from build123d import *

# Parameters (mm, degrees)
F0_R     = 1.5
F1_DEPTH = 1
F3_DEPTH = 25


with BuildPart() as f1:
    # F0 (on Top) → F1 (new body)
    with BuildSketch(Plane.XY):
        Polygon((125, -216.506351), (250, 0), (125, 216.506351), (-125, 216.506351), (-250, 0), (-125, -216.506351), align=None)
        with Locations((-153.300327, -114.488747)):
            Circle(F0_R, mode=Mode.SUBTRACT)
        with Locations((-22.5, -190.006351)):
            Circle(F0_R, mode=Mode.SUBTRACT)
        with Locations((-22.5, -174.006351)):
            Circle(F0_R, mode=Mode.SUBTRACT)
        with Locations((-139.44392, -106.488747)):
            Circle(F0_R, mode=Mode.SUBTRACT)
        with Locations((-175.800327, -75.517604)):
            Circle(F0_R, mode=Mode.SUBTRACT)
        with Locations((-161.94392, -67.517604)):
            Circle(F0_R, mode=Mode.SUBTRACT)
        with Locations((-66.697786, -64.488747)):
            Circle(F0_R, mode=Mode.SUBTRACT)
        with Locations((-22.5, -90.006351)):
            Circle(F0_R, mode=Mode.SUBTRACT)
        with Locations((-52.84138, -56.488747)):
            Circle(F0_R, mode=Mode.SUBTRACT)
        with Locations((-22.5, -74.006351)):
            Circle(F0_R, mode=Mode.SUBTRACT)
        with Locations((-89.197786, -25.517604)):
            Circle(F0_R, mode=Mode.SUBTRACT)
        with Locations((-75.34138, -17.517604)):
            Circle(F0_R, mode=Mode.SUBTRACT)
        with Locations((22.5, -190.006351)):
            Circle(F0_R, mode=Mode.SUBTRACT)
        with Locations((22.5, -174.006351)):
            Circle(F0_R, mode=Mode.SUBTRACT)
        with Locations((153.300327, -114.488747)):
            Circle(F0_R, mode=Mode.SUBTRACT)
        with Locations((22.5, -90.006351)):
            Circle(F0_R, mode=Mode.SUBTRACT)
        with Locations((22.5, -74.006351)):
            Circle(F0_R, mode=Mode.SUBTRACT)
        with Locations((52.84138, -56.488747)):
            Circle(F0_R, mode=Mode.SUBTRACT)
        with Locations((66.697786, -64.488747)):
            Circle(F0_R, mode=Mode.SUBTRACT)
        with Locations((75.34138, -17.517604)):
            Circle(F0_R, mode=Mode.SUBTRACT)
        with Locations((89.197786, -25.517604)):
            Circle(F0_R, mode=Mode.SUBTRACT)
        with Locations((139.44392, -106.488747)):
            Circle(F0_R, mode=Mode.SUBTRACT)
        with Locations((175.800327, -75.517604)):
            Circle(F0_R, mode=Mode.SUBTRACT)
        with Locations((161.94392, -67.517604)):
            Circle(F0_R, mode=Mode.SUBTRACT)
        with Locations((-161.94392, 67.517604)):
            Circle(F0_R, mode=Mode.SUBTRACT)
        with Locations((-175.800327, 75.517604)):
            Circle(F0_R, mode=Mode.SUBTRACT)
        with Locations((-139.44392, 106.488747)):
            Circle(F0_R, mode=Mode.SUBTRACT)
        with Locations((-89.197786, 25.517604)):
            Circle(F0_R, mode=Mode.SUBTRACT)
        with Locations((-75.34138, 17.517604)):
            Circle(F0_R, mode=Mode.SUBTRACT)
        with Locations((-66.697786, 64.488747)):
            Circle(F0_R, mode=Mode.SUBTRACT)
        with Locations((-52.84138, 56.488747)):
            Circle(F0_R, mode=Mode.SUBTRACT)
        with Locations((-22.5, 74.006351)):
            Circle(F0_R, mode=Mode.SUBTRACT)
        with Locations((-22.5, 90.006351)):
            Circle(F0_R, mode=Mode.SUBTRACT)
        with Locations((-153.300327, 114.488747)):
            Circle(F0_R, mode=Mode.SUBTRACT)
        with Locations((-22.5, 174.006351)):
            Circle(F0_R, mode=Mode.SUBTRACT)
        with Locations((-22.5, 190.006351)):
            Circle(F0_R, mode=Mode.SUBTRACT)
        with Locations((75.34138, 17.517604)):
            Circle(F0_R, mode=Mode.SUBTRACT)
        with Locations((89.197786, 25.517604)):
            Circle(F0_R, mode=Mode.SUBTRACT)
        with Locations((22.5, 74.006351)):
            Circle(F0_R, mode=Mode.SUBTRACT)
        with Locations((52.84138, 56.488747)):
            Circle(F0_R, mode=Mode.SUBTRACT)
        with Locations((22.5, 90.006351)):
            Circle(F0_R, mode=Mode.SUBTRACT)
        with Locations((66.697786, 64.488747)):
            Circle(F0_R, mode=Mode.SUBTRACT)
        with Locations((161.94392, 67.517604)):
            Circle(F0_R, mode=Mode.SUBTRACT)
        with Locations((175.800327, 75.517604)):
            Circle(F0_R, mode=Mode.SUBTRACT)
        with Locations((139.44392, 106.488747)):
            Circle(F0_R, mode=Mode.SUBTRACT)
        with Locations((22.5, 174.006351)):
            Circle(F0_R, mode=Mode.SUBTRACT)
        with Locations((22.5, 190.006351)):
            Circle(F0_R, mode=Mode.SUBTRACT)
        with Locations((153.300327, 114.488747)):
            Circle(F0_R, mode=Mode.SUBTRACT)
    extrude(amount=F1_DEPTH)

    # F2 (on face) → F3 (cut)
    with BuildSketch(Plane.XY.offset(1)):
        Polygon((-110.432692, 196.217343), (-144.11898, 134.459153), (-60.60506, 85.333318), (-43.761913, 100.772865), (-43.761913, 196.217343), align=None)
        Polygon((-225.14555, 2.471155), (-188.504532, -57.581121), (-104.203351, -9.818863), (-109.152818, 12.487504), (-191.81016, 60.209743), align=None)
        Polygon((-114.712858, -193.746188), (-44.385552, -192.040274), (-43.598291, -95.152181), (-65.390905, -88.285361), (-148.048248, -136.0076), align=None)
        Polygon((110.432692, -196.217343), (144.11898, -134.459153), (60.60506, -85.333318), (43.761913, -100.772865), (43.761913, -196.217343), align=None)
        Polygon((225.14555, -2.471155), (188.504532, 57.581121), (104.203351, 9.818863), (109.152818, -12.487504), (191.81016, -60.209743), align=None)
        Polygon((114.712858, 193.746188), (44.385552, 192.040274), (43.598291, 95.152181), (65.390905, 88.285361), (148.048248, 136.0076), align=None)
    extrude(amount=-F3_DEPTH, mode=Mode.SUBTRACT)


solid = f1.part
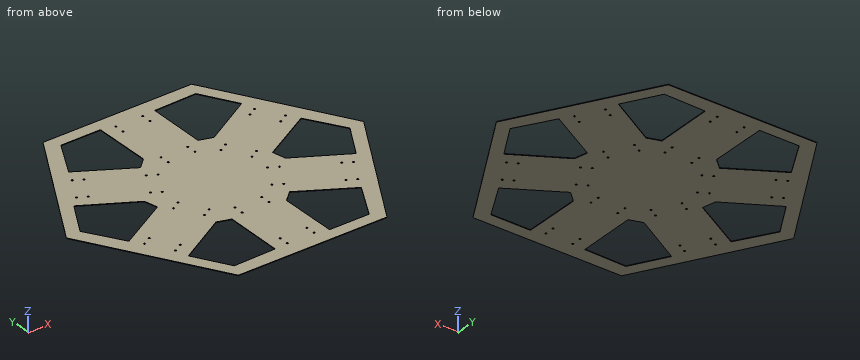
Can you work these out from the model? Positions are in its coordinate system, mm. Coordinates: 2 decimals unless noted, no trailing zeros. Write each loop counter-clockwise with the first axis right and the second up, starting at its lowest first coordinate (ties: lowest second). Pieces come first, ordered by that corner, then holes. Notation, with made-up numbers: (64.5, 25.5) -> (81.5, 25.5) arc R18 cw to (81.5, 43.5) -> close; hole circle Ø11 at (-5.5, -38.75). An arc over 180 degrees is marked (long way). Write each question's results on one line, items separated by ' | '. Start each with the question number.
Item 1: If we section it at A-A, the plane y = -141.5: Write out the boundary of the cut face in (x, z).
Item 2: Please list where these lines run through material, in increasing order: probe 1 along Y at (x, z) = (-59, 0.7); probe 2 along X at (y, z) = (76, 0.65); probe 3 along X at (y, z) = (-27.5, 0.7).
Item 3: If we section it at B-B, the plane z = 0.45: Count the separate pieces of the cut face and the enclosed holes in it, and give its area (3 significant figures).
Answer block:
1) outline: (-168.3, 0) -> (-144.88, 0) -> (-144.88, 1) -> (-168.3, 1) -> close; (-43.97, 0) -> (43.76, 0) -> (43.76, 1) -> (-43.97, 1) -> close; (140.28, 0) -> (168.3, 0) -> (168.3, 1) -> (140.28, 1) -> close
2) probe 1: -216.51 to -192.39, -90.3 to 86.8, 196.22 to 216.51 | probe 2: -206.12 to -177.22, -174.38 to 174.38, 177.22 to 206.12 | probe 3: -234.12 to -206.86, -135.41 to 135.16, 210.7 to 234.12
3) separate pieces: 1 | enclosed holes: 54 | area: 115,000 mm²
